Could you check a few things on this drawing? It's one solid part, dimensions in mm from its lowest x, y, z. A direction names the side the tool comes from. Give positions to 0.01 mm unless a question says otherwise; leave off trailing zeros. Order: outer loops, then holes, each group sorted by start corner. A loop starts at its lowest first (then second) coordinate and runs counter-clockwise, first axis right, second up.
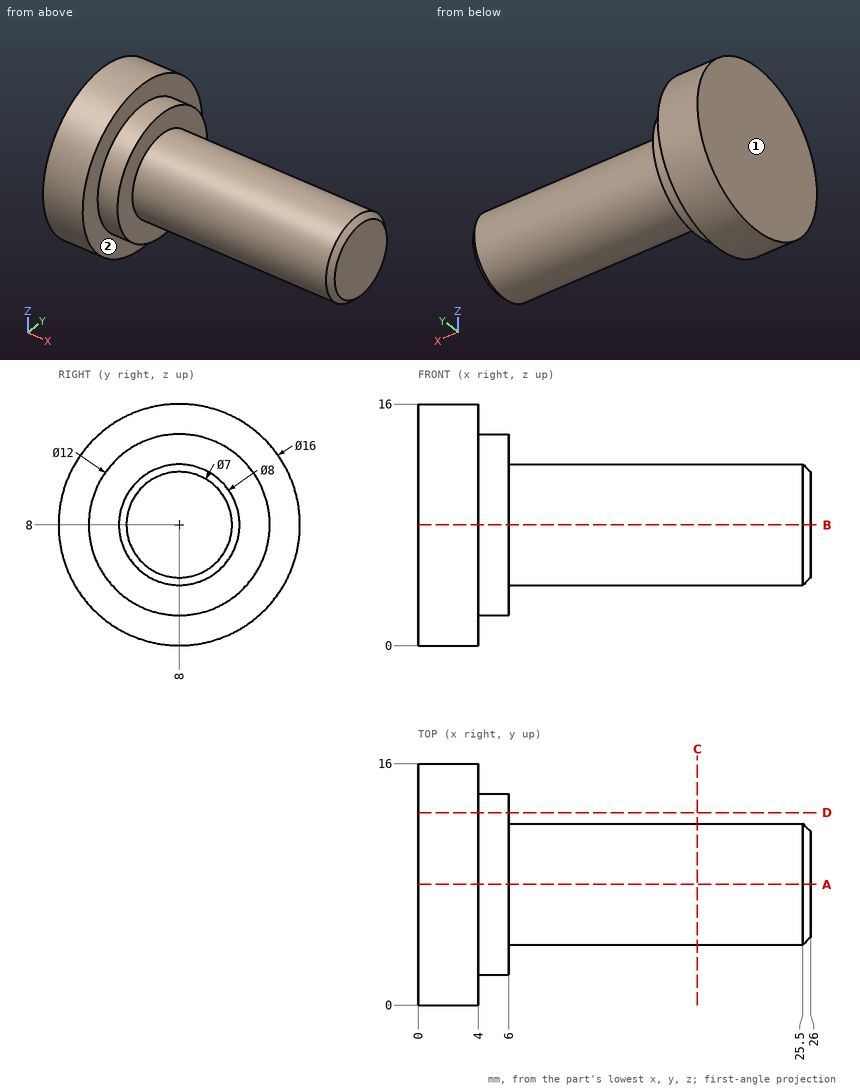
Q1. If we section it at A-A on y = 8: List the corners of the cut face in (x, z) for me, plus the area to 3 significant figures.
Filled sheet:
outline: (0, 0) - (4, 0) - (4, 2) - (6, 2) - (6, 4) - (25.5, 4) - (26, 4.5) - (26, 11.5) - (25.5, 12) - (6, 12) - (6, 14) - (4, 14) - (4, 16) - (0, 16) - close
area: 248 mm2
Q2. I need wall thicknesses on L1, parallel to X at y = 4.75, z = 1; L2, parallel to X at y = 12.5, z = 7.5; L3, parallel to Z at x = 3.25, y = 12.5. Which ranges of each line are inside material? Lowest first, please.
Filled sheet:
L1: x = 0 to 4
L2: x = 0 to 6
L3: z = 1.39 to 14.61
Q3. If we section it at D-D on y = 12.75: List the corners of the cut face in (x, z) for me.
Filled sheet:
outline: (0, 1.56) - (4, 1.56) - (4, 4.33) - (6, 4.33) - (6, 11.67) - (4, 11.67) - (4, 14.44) - (0, 14.44) - close
Q4. If we section it at C-C on x = 18.5: List the corners of the cut face in (y, z) for me, plus the area to 3 significant figures.
Filled sheet:
outline: circle Ø8 at (8, 8)
area: 50.3 mm2
Q5. I'm going to push flat-ended pins straight in: P1, Ø1.5, axis at x = 7.5, z = 6.5, coming from the +Y side; P2, Ø5, axis at x = 16, y = 3.5, coming from the -Z side; P3, Ø1, axis at y = 9, z = 13, coming from the +X side. Where does each tip first touch, or does it pass through?
Filled sheet:
P1: stops at y = 11.93
P2: stops at z = 4.54
P3: stops at x = 6
Q6. For the marked faces 1 and 2, which set-ups out of +Z, -Z, +X, -X, +Y, -Y let a thin tool reach every point of the face, with its end or its side?
Filled sheet:
face 1: +Z, -Z, -X, +Y, -Y
face 2: +X
